Verification items for the finished model (mm, model axes). Face numbers are marked on the shaded views. A direction names the side the tool comes from. Give positions to 0.01 mm unless a question says otherwise; leave off trailing zeros. Order: outer loops, then holes, each group sorted by start corner. A loop starts at its lowest first (then second) coordinate and runs counter-clockwise, first axis right, second up. Notation, with made-up numbers: (-8.5, 76) -> (-0.5, 76) arc R20 cw to (-0.5, 97) -> close; hole circle Ø1 at (-15.75, -35.5). An arc over 180 degrees is marked (long way). Return JSON: item names as keys, results as strings. Group by question number.
(1) Tool access check on the marked faces 1, 2, 3 and 4. Record the directions out of +Z, -Z, +X, -X, +Y, -Y that give a thin tool (end or side, any length) a straight path to the whole face; none if there is none.
(2) Cross-section at C-C on z = -30. Enter the section's corners in (x, y), then the cut area to 3 significant figures.
(3) Release check for a two-part mould opening along Y. For the marked faces 5, 6 and 7 record: pulls with the +Y half, pulls with the -Y half, needs draft (parallel to the pull), parting line crosses it, or undercut.
(4) Thickness scan on line 1 along Y through (x, z) = (16, -43.75); line 2 along X through (y, z) = (17.5, -40.5); line 3 along Y through (x, z) = (7.5, -9). Record the ranges inside material, lowest first.
(5) Cross-section at B-B on y = 13. State how many separate pieces and enclosed holes the cut face has, then the cut area to 3 significant figures.
(6) Cross-section at A-A on x = -63.5. Enter the section's corners in (y, z).
(7) Depth check by flat-ended pin: pin 1 Ø1 at (y, z) = (19.5, -13.5) entering from -X; pin 2 Ø6.5 at (x, z) = (15.5, 8) entering from +Y; pin 3 Ø1 at (x, z) = (-57, 3.5) entering from -Y; pin 4 Ø2.5 at (y, z) = (22, -18) entering from -X. Enter the tip coordinate at first touch or a pass-through.
from build123d import *

# Parameters (mm, degrees)
SKETCH_1_R           = 1.7
SKETCH_1_R_2         = 5.4
EXTRUDE_1_DEPTH      = 10
EXTRUDE_START        = -10
EXTRUDE_2_DEPTH      = 10
CUT_EXTRUDE_1_DEPTH  = 2
EXTRUDE_START_2      = -46
EXTRUDE_3_DEPTH      = 36
EXTRUDE_START_3      = 6.5
EXTRUDE_4_DEPTH      = 3.5
EXTRUDE_5_DEPTH      = 4
SKETCH_1_10_W        = 8
SKETCH_1_10_H        = 8
SKETCH_1_10_R        = 1.5
EXTRUDE_6_DEPTH      = 7
RIB_2_REACH          = 105.331
SKETCH_4_WALL_W      = 219.975267576
SKETCH_4_WALL_H      = 1
RIB_START            = -1
RIB_3_DEPTH          = 1
EXTRUDE_START_4      = -0.4
SKETCH_6_R           = 1.5
EXTRUDE_7_DEPTH      = 0.4
SKETCH_7_R           = 1.7
SKETCH_7_R_2         = 1.35
CUT_EXTRUDE_2_DEPTH  = 89.290712988
SKETCH_8_W           = 26
SKETCH_8_H           = 10
CUT_EXTRUDE_3_DEPTH  = 105.174133066
CUT_EXTRUDE_4_DEPTH  = 22
CUT_EXTRUDE_5_DEPTH  = 24
SKETCH_7_4_W         = 2.4
SKETCH_7_4_H         = 10
CUT_EXTRUDE_9_DEPTH  = 15.05
CHAMFER_1_SIZE       = 3.7
CUT_EXTRUDE_START    = -17.562916
SKETCH_7_5_W         = 3
SKETCH_7_5_H         = 6
CUT_EXTRUDE_10_DEPTH = 17.562916
CUT_EXTRUDE_11_REACH = 90.291
CHAMFER_2_SIZE       = 5
CHAMFER_3_SIZE       = 2
CHAMFER_3_SIZE2      = 2.5
SKETCH_9_W           = 11.322924712
SKETCH_9_H           = 24.282583949
CUT_EXTRUDE_12_DEPTH = 93.82914413


# Read off the part's stored shape, not the designer's step: 筋3
with BuildPart() as part:
    # 草图1 → 凸台-拉伸1 (new body)
    with BuildSketch(Plane.XY):
        with BuildLine():
            Line((-17, -7.5), (-17, -11))
            Line((-17, -11), (0, -11))
            ThreePointArc((0, -11), (7.778174593, -7.778174593), (11, 0))
            Line((11, 0), (11, 8.456854249))
            Line((11, 8.456854249), (28, 8.456854249))
            Line((28, 8.456854249), (28, 10.5))
            Line((28, 10.5), (21, 10.5))
            Line((21, 10.5), (21, 20.5))
            Line((21, 20.5), (28, 20.5))
            Line((28, 20.5), (28, 23.5))
            Line((28, 23.5), (-67, 23.5))
            Line((-67, 23.5), (-67, 7.5))
            Line((-67, 7.5), (-17, 7.5))
            ThreePointArc((-17, 7.5), (-9.5, 0), (-17, -7.5))
        make_face()
        with Locations((-5.656854249, -5.656854249)):
            Circle(SKETCH_1_R, mode=Mode.SUBTRACT)
        with Locations((5.656854249, -5.656854249)):
            Circle(SKETCH_1_R, mode=Mode.SUBTRACT)
        Circle(SKETCH_1_R_2, mode=Mode.SUBTRACT)
        with Locations((-5.656854249, 5.656854249)):
            Circle(SKETCH_1_R, mode=Mode.SUBTRACT)
        with Locations((5.656854249, 5.656854249)):
            Circle(SKETCH_1_R, mode=Mode.SUBTRACT)
    extrude(amount=EXTRUDE_1_DEPTH)

    # 草图1<6> → 凸台-拉伸2 (add)
    with BuildSketch(Plane.XY.offset(EXTRUDE_START)):
        with BuildLine():
            Line((21, 10.5), (21, 20.5))
            Line((21, 20.5), (28, 20.5))
            Line((28, 20.5), (28, 23.5))
            Line((28, 23.5), (-67, 23.5))
            Line((-67, 23.5), (-67, 7.5))
            Line((-67, 7.5), (-17, 7.5))
            ThreePointArc((-17, 7.5), (-9.5, 0), (-17, -7.5))
            Line((-17, -7.5), (-17, -11))
            ThreePointArc((-17, -11), (-8.462447466, -5.036106671), (-8.643737412, 5.376624039))
            ThreePointArc((-8.643737412, 5.376624039), (-7.46899014, 8.047704206), (-4.579821288, 8.456854249))
            Line((-4.579821288, 8.456854249), (28, 8.456854249))
            Line((28, 8.456854249), (28, 10.5))
            Line((28, 10.5), (21, 10.5))
        make_face()
    extrude(amount=EXTRUDE_2_DEPTH)

    # 草图3 → 切除-拉伸1 (cut)
    with BuildSketch(Plane(origin=(0, 0, 0), x_dir=(-1, 0, 0), z_dir=(0, 0, -1))):
        Polygon((7.919595949, 3.39411255), (8.747816894, 6.485075194), (6.485075194, 8.747816894), (3.39411255, 7.919595949), (2.565891605, 4.828633305), (4.828633305, 2.565891605), align=None)
        Polygon((-2.565891605, 4.828633305), (-3.39411255, 7.919595949), (-6.485075194, 8.747816894), (-8.747816894, 6.485075194), (-7.919595949, 3.39411255), (-4.828633305, 2.565891605), align=None)
        Polygon((-3.39411255, -7.919595949), (-2.565891605, -4.828633305), (-4.828633305, -2.565891605), (-7.919595949, -3.39411255), (-8.747816894, -6.485075194), (-6.485075194, -8.747816894), align=None)
        Polygon((2.565891605, -4.828633305), (3.39411255, -7.919595949), (6.485075194, -8.747816894), (8.747816894, -6.485075194), (7.919595949, -3.39411255), (4.828633305, -2.565891605), align=None)
    extrude(amount=-CUT_EXTRUDE_1_DEPTH, mode=Mode.SUBTRACT)

    # 草图1<7> → 凸台-拉伸3 (add)
    with BuildSketch(Plane.XY.offset(EXTRUDE_START_2)):
        with BuildLine():
            Line((21, 8.456854249), (21, 23.5))
            Line((21, 23.5), (-67, 23.5))
            Line((-67, 23.5), (-67, 7.5))
            Line((-67, 7.5), (-17, 7.5))
            ThreePointArc((-17, 7.5), (-9.5, 0), (-17, -7.5))
            Line((-17, -7.5), (-17, -11))
            ThreePointArc((-17, -11), (-8.462447466, -5.036106671), (-8.643737412, 5.376624039))
            ThreePointArc((-8.643737412, 5.376624039), (-7.46899014, 8.047704206), (-4.579821288, 8.456854249))
            Line((-4.579821288, 8.456854249), (21, 8.456854249))
        make_face()
    extrude(amount=EXTRUDE_3_DEPTH)

    # 草图1<8> → 凸台-拉伸4 (add)
    with BuildSketch(Plane.XY.offset(EXTRUDE_START_3)):
        with BuildLine():
            Line((-17, -5), (-17, -7.5))
            ThreePointArc((-17, -7.5), (-9.5, 0), (-17, 7.5))
            Line((-17, 7.5), (-17, 5))
            ThreePointArc((-17, 5), (-12, 0), (-17, -5))
        make_face()
    extrude(amount=EXTRUDE_4_DEPTH)

    # 草图1<9> → 凸台-拉伸5 (add)
    with BuildSketch(Plane.XY.offset(EXTRUDE_START_2)):
        with BuildLine():
            Line((-17, -5), (-17, -7.5))
            ThreePointArc((-17, -7.5), (-9.5, 0), (-17, 7.5))
            Line((-17, 7.5), (-17, 5))
            ThreePointArc((-17, 5), (-12, 0), (-17, -5))
        make_face()
    extrude(amount=EXTRUDE_5_DEPTH)

    # 草图1<10> → 凸台-拉伸6 (add)
    with BuildSketch(Plane.XY.offset(EXTRUDE_START_2)):
        with Locations((16, 27.5)):
            Rectangle(SKETCH_1_10_W, SKETCH_1_10_H)
        with Locations((16, 27.5)):
            Circle(SKETCH_1_10_R, mode=Mode.SUBTRACT)
    extrude(amount=EXTRUDE_6_DEPTH)

    # 草图4 wall → 筋2 (add, up to next)
    with BuildSketch(Plane(origin=(20, 27.5, -35), x_dir=(0, -0.707106781187, 0.707106781187), z_dir=(0, -0.707106781187, -0.707106781187)), mode=Mode.PRIVATE) as rib_2_sk1:
        with Locations((0, 0.5)):
            Rectangle(SKETCH_4_WALL_W, SKETCH_4_WALL_H)
    rib_2_tool1 = extrude(rib_2_sk1.sketch, amount=RIB_2_REACH, mode=Mode.PRIVATE) - part.part
    add(rib_2_tool1.solids().sort_by_distance((20, 27.5, -35))[0])

    # 筋3 outline → 筋3 (add)
    with BuildSketch(Plane.ZY.offset(-12).offset(RIB_START)):
        Polygon((-31, 23.5), (-39, 31.5), (-39, 23.5), align=None)
    extrude(amount=RIB_3_DEPTH)

    # 草图6 → 凸台-拉伸7 (add)
    with BuildSketch(Plane.XY.offset(-39).offset(EXTRUDE_START_4)):
        with Locations((16, 27.5)):
            Circle(SKETCH_6_R)
    extrude(amount=EXTRUDE_7_DEPTH)

    # 草图7 → 切除-拉伸2 (cut, through all)
    with BuildSketch(Plane(origin=(0, 23.5, 0), x_dir=(1, 0, 0), z_dir=(0, 1, 0))):
        with BuildLine():
            Line((-17, 38), (-17, 46))
            Line((-17, 46), (-69, 46))
            Line((-69, 46), (-69, 5))
            Line((-69, 5), (-48, 5))
            ThreePointArc((-48, 5), (-38.807611845, 8.807611845), (-35, 18))
            Line((-35, 18), (-35, 38))
            Line((-35, 38), (-17, 38))
        make_face()
        with Locations(Location((12.7, 18, 0), (0, 0, 180))):
            Circle(SKETCH_7_R)
        with Locations(Location((16, -6, 0), (0, 0, 180))):
            Circle(SKETCH_7_R)
        with Locations(Location((8, 42, 0), (0, 0, 180))):
            Circle(SKETCH_7_R)
        with Locations(Location((-32.5, 2.5, 0), (0, 0, 180))):
            Circle(SKETCH_7_R)
        with Locations(Location((-63.5, 2.5, 0), (0, 0, 180))):
            Circle(SKETCH_7_R)
        with Locations(Location((-32.5, 33.5, 0), (0, 0, 180))):
            Circle(SKETCH_7_R)
        with Locations(Location((24.5, -5, 0), (0, 0, 180))):
            Circle(SKETCH_7_R_2)
        with Locations(Location((24.5, 5, 0), (0, 0, 270))):
            Circle(SKETCH_7_R_2)
    extrude(amount=-CUT_EXTRUDE_2_DEPTH, mode=Mode.SUBTRACT)

    # 草图8 → 切除-拉伸3 (cut, through all)
    with BuildSketch(Plane(origin=(21, 0, 0), x_dir=(0, 0, -1), z_dir=(1, 0, 0))):
        with Locations((18, 15.5)):
            Rectangle(SKETCH_8_W, SKETCH_8_H)
    extrude(amount=-CUT_EXTRUDE_3_DEPTH, mode=Mode.SUBTRACT)

    # 草图8<3> → 切除-拉伸4 (cut)
    with BuildSketch(Plane(origin=(21, 0, 0), x_dir=(0, 0, -1), z_dir=(1, 0, 0))):
        with BuildLine():
            ThreePointArc((36, 19.7), (31.8, 15.5), (36, 11.3))
            Line((36, 11.3), (36, 19.7))
        make_face()
        with BuildLine():
            ThreePointArc((4.2, 15.5), (2.969848481, 18.469848481), (0, 19.7))
            Line((0, 19.7), (0, 11.3))
            ThreePointArc((0, 11.3), (2.969848481, 12.530151519), (4.2, 15.5))
        make_face()
    extrude(amount=-CUT_EXTRUDE_4_DEPTH, mode=Mode.SUBTRACT)

    # 草图8<4> → 切除-拉伸5 (cut)
    with BuildSketch(Plane(origin=(21, 0, 0), x_dir=(0, 0, -1), z_dir=(1, 0, 0))):
        with BuildLine():
            Line((0, 11.3), (0, 19.7))
            ThreePointArc((0, 19.7), (-2.787471973, 18.641655614), (-4.170131892, 16))
            Line((-4.170131892, 16), (-10, 16))
            Line((-10, 16), (-10, 15))
            Line((-10, 15), (-4.170131892, 15))
            ThreePointArc((-4.170131892, 15), (-2.787471973, 12.358344386), (0, 11.3))
        make_face()
        with BuildLine():
            Line((40.170131892, 15), (46, 15))
            Line((46, 15), (46, 16))
            Line((46, 16), (40.170131892, 16))
            ThreePointArc((40.170131892, 16), (38.787471973, 18.641655614), (36, 19.7))
            Line((36, 19.7), (36, 11.3))
            ThreePointArc((36, 11.3), (38.787471973, 12.358344386), (40.170131892, 15))
        make_face()
    extrude(amount=-CUT_EXTRUDE_5_DEPTH, mode=Mode.SUBTRACT)

    # 草图7<4> → 切除-拉伸9 (cut)
    with BuildSketch(Plane(origin=(0, 23.5, 0), x_dir=(1, 0, 0), z_dir=(0, 1, 0))):
        with Locations((-2.2, -5)):
            Rectangle(SKETCH_7_4_W, SKETCH_7_4_H)
        with Locations((-2.2, 41)):
            Rectangle(SKETCH_7_4_W, SKETCH_7_4_H)
    extrude(amount=-CUT_EXTRUDE_9_DEPTH, mode=Mode.SUBTRACT)

    # 倒角1
    chamfer_1_edges = [part.edges().sort_by_distance(p)[0] for p in [
        (-1, 16, -43.085065946),
        (-1, 15, -43.085065946),
        (-1, 16, 7.085065946),
        (-1, 15, 7.085065946),
    ]]
    chamfer(chamfer_1_edges, length=CHAMFER_1_SIZE)

    # 草图7<5> → 切除-拉伸10 (cut)
    with BuildSketch(Plane(origin=(0, 23.5, 0), x_dir=(1, 0, 0), z_dir=(0, 1, 0)).offset(CUT_EXTRUDE_START)):
        with Locations((-7.143737412, 18)):
            Rectangle(SKETCH_7_5_W, SKETCH_7_5_H)
        with Locations((-7.143737412, 28)):
            Rectangle(SKETCH_7_5_W, SKETCH_7_5_H)
        with Locations((-23, 28)):
            Rectangle(SKETCH_7_5_W, SKETCH_7_5_H)
        with Locations((-23, 18)):
            Rectangle(SKETCH_7_5_W, SKETCH_7_5_H)
        with Locations((-23, 8)):
            Rectangle(SKETCH_7_5_W, SKETCH_7_5_H)
        with Locations((-7.143737412, 8)):
            Rectangle(SKETCH_7_5_W, SKETCH_7_5_H)
    extrude(amount=CUT_EXTRUDE_10_DEPTH, mode=Mode.SUBTRACT)

    # 草图7<6> → 切除-拉伸11 (cut, up to next)
    with BuildSketch(Plane(origin=(0, 23.5, 0), x_dir=(1, 0, 0), z_dir=(0, 1, 0)), mode=Mode.PRIVATE) as cut_extrude_11_sk1:
        Polygon((-21.5, 5), (-8.643737412, 5), (-8.643737412, 11), (-5.643737412, 11), (-5.643737412, 15), (-8.643737412, 15), (-8.643737412, 21), (-5.643737412, 21), (-5.643737412, 25), (-8.643737412, 25), (-8.643737412, 31), (-21.5, 31), (-21.5, 25), (-24.5, 25), (-24.5, 21), (-21.5, 21), (-21.5, 15), (-24.5, 15), (-24.5, 11), (-21.5, 11), align=None)
    cut_extrude_11_tool1 = extrude(cut_extrude_11_sk1.sketch, amount=-CUT_EXTRUDE_11_REACH, mode=Mode.PRIVATE) & part.part
    add(cut_extrude_11_tool1.solids().sort_by_distance((-15.071869, 23.5, -18))[0], mode=Mode.SUBTRACT)

    # 倒角2
    chamfer_2_edges = [part.edges().sort_by_distance(p)[0] for p in [
        (-5.643737412, 22, -31),
        (-24.5, 22, -31),
    ]]
    chamfer(chamfer_2_edges, length=CHAMFER_2_SIZE)

    # 倒角3
    chamfer_3_edges = [part.edges().sort_by_distance(p)[0] for p in [
        (-12, 0, -42),
    ]]
    chamfer_3_side = [part.faces().sort_by_distance(p)[0] for p in [
        (-9.667705098, 0, -42),
    ]]
    chamfer(chamfer_3_edges, length=CHAMFER_3_SIZE, length2=CHAMFER_3_SIZE2, reference=chamfer_3_side[0])

    # 草图9 → 切除-拉伸12 (cut, through all)
    with BuildSketch(Plane.XY.offset(10)):
        with Locations((25.661462356, 19.358708026)):
            Rectangle(SKETCH_9_W, SKETCH_9_H)
    extrude(amount=-CUT_EXTRUDE_12_DEPTH, mode=Mode.SUBTRACT)


solid = part.part
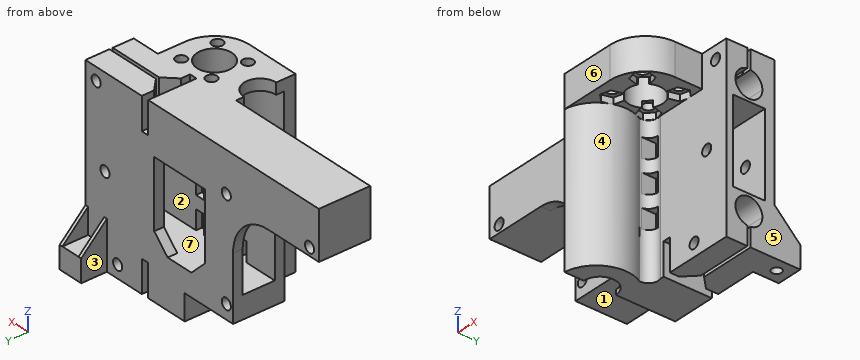
Verdict:
{
 "1": {"face 1": "-Z, -X, +Y, -Y", "face 2": "+X, -X", "face 3": "+Z, -Z, -X, +Y", "face 4": "-Z, +X"},
 "2": {"outline": "(-35, 7.5) -> (-24.5, 7.5) -> (-24.5, 10.5) -> (-35, 10.5) -> close; (-35, 20.5) -> (-20.5, 20.5) -> (-20.5, 23.5) -> (-35, 23.5) -> close; (-21.5, 7.5) -> (-17, 7.5) arc R7.5 cw to (-17, -7.5) -> (-17, -11) arc R11.08 ccw to (-8.64, 5.38) arc R3 cw to (-8.64, 5.94) -> (-8.64, 10.5) -> (-21.5, 10.5) -> close; (-9.64, 20.5) -> (20, 20.5) -> (20, 23.5) -> (-9.64, 23.5) -> close; (-5.64, 8.66) arc R3 cw to (-4.58, 8.46) -> (20, 8.46) -> (20, 10.5) -> (-5.64, 10.5) -> close", "area": "316 mm²"},
 "3": {"face 5": "needs draft", "face 6": "pulls with the -Y half", "face 7": "undercut"},
 "4": {"line 1": "8.46 to 15, 16 to 26, 29 to 31.5", "line 2": "-17 to -3.4, 1.2 to 7.2, 8.8 to 20", "line 3": "8.46 to 10.5, 20.5 to 23.5"},
 "5": {"separate pieces": "4", "enclosed holes": "5", "area": "1,590 mm²"},
 "6": {"outline": "(7.5, -5) -> (23.5, -5) -> (23.5, -4.2) -> (7.5, -4.2) -> close; (7.5, -0.8) -> (23.5, -0.8) -> (23.5, 10) -> (7.5, 10) -> close"},
 "7": {"pin 1": "through", "pin 2": "y = 23.5", "pin 3": "y = 7.5", "pin 4": "x = -35.06"}
}
